Read the model definition and answer for the solid it produces. Units are mm, in the model's axes. A direction names the side the tool comes from. Coordinates: 2 decimals unless noted, no trailing zeros. Order: outer loops, then holes, each group sorted by start corner. A loop starts at its lowest first (then second) coordinate and runs counter-clockwise, first axis right, second up. Notation, with made-up numbers: M 67.25,-1 L 118.25,-1 A13 cw 118.25,13 Z; hole C -18.5,32.25 d11. An arc over 180 degrees is marked long. Write each question's results on one line, items separated by ' | '.
```python
from build123d import *

# Parameters (mm, degrees)
FILLET1_R               = 2
SKETCH2_R               = 5
CUT_EXTRUDE1_DEPTH      = 16
CUT_EXTRUDE1_DEPTH_BACK = 16


with BuildPart() as part:
    # Sketch1 → Revolve1 (revolve)
    with BuildSketch(Plane.XY):
        Polygon((-782.772277228, 0), (-782.772277228, 15), (2.227722772, 15), (2.227722772, 11.732673267), (32.227722772, 11.732673267), (57.227722772, 7.5), (77.227722772, 7.5), (77.227722772, 0), align=None)
    revolve(axis=Axis((-782.772277228, 0, 0), (1, 0, 0)))

    # Fillet1
    fillet1_edges = [part.edges().sort_by_distance(p)[0] for p in [
        (2.227722772, -15, 0),
    ]]
    fillet(fillet1_edges, radius=FILLET1_R)

    # Sketch2 → Cut-Extrude1 (cut, two sides)
    with BuildSketch(Plane.XY) as cut_extrude1_sk:
        with Locations((-522.772277228, 0)):
            Circle(SKETCH2_R)
        with Locations((-282.772277228, 0)):
            Circle(SKETCH2_R)
    extrude(amount=CUT_EXTRUDE1_DEPTH, mode=Mode.SUBTRACT)
    extrude(cut_extrude1_sk.sketch, amount=-CUT_EXTRUDE1_DEPTH_BACK, mode=Mode.SUBTRACT)


solid = part.part
```
(1) The part is cut by section A-A, the plane y = 0. Write down the section's boundary in (x, z), then the cut area to 3 significant figures.
Conclusion:
outline: M -782.77,-15 L -527.77,-15 L -527.77,15 L -782.77,15 Z; M -517.77,-15 L -287.77,-15 L -287.77,15 L -517.77,15 Z; M -277.77,-15 L 0.23,-15 A2 ccw 2.23,-13 L 2.23,-11.73 L 32.23,-11.73 L 57.23,-7.5 L 77.23,-7.5 L 77.23,7.5 L 57.23,7.5 L 32.23,11.73 L 2.23,11.73 L 2.23,13 A2 ccw 0.23,15 L -277.77,15 Z | area: 24,400 mm²
(2) For faces 1 (the cylindrical face through (-385.791, -14.985, 0.66)), 2 (the flat face through (2.228, -2, 12)), determine the directions among +Z, -Z, +X, -X, +Y, -Y from which every point of the face is accessible in a straight line to the end or side of a thin tool.
Conclusion:
face 1: +X, -X | face 2: +X
(3) Straight lines are drawn through the part: line 1 (X direction, y = 0, z = 6); line 2 (X direction, y = 4.5, z = 0); line 3 (Y direction, x = -199, z = -0.5). For each, find the intervals that lie inside material, in ascending order.
Conclusion:
line 1: -782.77 to -527.77, -517.77 to -287.77, -277.77 to 77.23 | line 2: -782.77 to -524.95, -520.59 to -284.95, -280.59 to 77.23 | line 3: -14.99 to 14.99
(4) Given pin 1 (4 mm diameter, centred on x = -152, z = 6.5, fed in from -Y); pin 2 (8 mm diameter, centred on x = -282.77, y = 0, fed in from -Z); pin 3 (5 mm diameter, centred on x = -538, z = 8, fed in from +Y); pin 4 (5 mm diameter, centred on x = -91, z = 5, fed in from -Y), each flat-ended and moving along its own axis, determine where each tip first touches the part or whether it passes through.
Conclusion:
pin 1: y = -14.31 | pin 2: through | pin 3: y = 13.96 | pin 4: y = -14.79
(5) The part is cut by section B-B, the plane x = -84.5. Write down the section's boundary in (y, z), then the cut area to 3 significant figures.
Conclusion:
outline: C 0,0 d30 | area: 707 mm²
